The listing builds one solid part. Answer for the finished solid, in the listing's coordinates (mm). Face numbers are marked on the shaded views. A direction names the side the tool comes from. Round coordinates to 2 decimals unless told otherwise and drop trailing zeros. Loops run counter-clockwise (first coordinate to the right, second up) from the corner with the lowest first, then second, coordinate; pieces in that order, holes last. Notation, with made-up numbers: (30.25, 17.25) -> (76.25, 17.25) arc R17 ccw to (76.25, 38.25) -> close; hole circle Ø2 at (26.5, -15.5). An arc over 180 degrees is marked (long way). Answer in a Markdown table with one row per item. Add a question column.
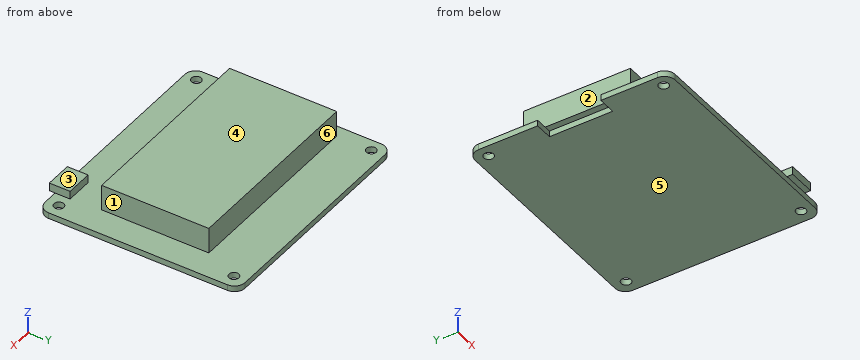
```python
from build123d import *

# Parameters (mm, degrees)
SKETCH_R     = 1.375
PAD_DEPTH    = 1.65
SKETCH001_W  = 54
SKETCH001_H  = 30
PAD001_DEPTH = 7.2
SKETCH002_W  = 7.57
SKETCH002_H  = 5.81
PAD002_DEPTH = 2.25


with BuildPart() as part:
    # Sketch (on Face4 of Binder) → Pad (new body)
    with BuildSketch(Plane.XY.offset(10.5)):
        with BuildLine():
            Line((-48.266962, 27.485719), (-48.266962, 10.985719))
            Line((-43.266962, 10.985719), (-48.266962, 10.985719))
            Line((-43.266962, -6.711357), (-43.266962, 10.985719))
            Line((-48.266962, -6.711357), (-43.266962, -6.711357))
            Line((-48.266962, -6.711357), (-48.266967, -22.514281))
            ThreePointArc((-48.266967, -22.514281), (-47.388287, -24.635602), (-45.266967, -25.514281))
            Line((-45.266967, -25.514281), (13.733038, -25.514281))
            ThreePointArc((13.733038, -25.514281), (15.854358, -24.635602), (16.733038, -22.514281))
            Line((16.733038, -22.514281), (16.733038, 27.485719))
            ThreePointArc((16.733038, 27.485719), (15.854358, 29.607039), (13.733038, 30.485719))
            Line((13.733038, 30.485719), (-45.266962, 30.485719))
            ThreePointArc((-45.266962, 30.485719), (-47.388282, 29.607039), (-48.266962, 27.485719))
        make_face()
        with Locations((-44.941962, 26.910719)):
            Circle(SKETCH_R, mode=Mode.SUBTRACT)
        with Locations((13.058038, 26.910719)):
            Circle(SKETCH_R, mode=Mode.SUBTRACT)
        with Locations((13.058038, -22.089281)):
            Circle(SKETCH_R, mode=Mode.SUBTRACT)
        with Locations((-44.941962, -22.089281)):
            Circle(SKETCH_R, mode=Mode.SUBTRACT)
    extrude(amount=PAD_DEPTH)

    # Sketch001 (on Face18 of Pad) → Pad001 (join)
    with BuildSketch(Plane.XY.offset(12.15)):
        with Locations((-18.066962, 2.137181)):
            Rectangle(SKETCH001_W, SKETCH001_H)
    extrude(amount=PAD001_DEPTH)

    # Sketch002 (on Face5 of Pad001) → Pad002 (join)
    with BuildSketch(Plane.XY.offset(12.15)):
        with Locations((5.748038, -24.209281)):
            Rectangle(SKETCH002_W, SKETCH002_H)
    extrude(amount=PAD002_DEPTH)


solid = part.part
```
Item 1: For the marked faces 1, 2 and 3, determine the directions among +Z, -Z, +X, -X, +Y, -Y from which every point of the face is accessible in a straight line to the end or side of a thin tool.
Item 2: Section A-A, the plane z = 13.5 is taken. Write down the section's boundary in (x, y).
Item 3: Section C-C, the plane y = 1 is taken. Write down the section's boundary in (x, z).
Item 4: Section B-B, the plane x = -38.5 is taken. Write down the section's boundary in (y, z), and give its area (3 significant figures).
Item 5: Flat-ended cylindrical pins translate along their axes: P1, Ø1, axis at x = 8, y = -21, coming from the +Z side; P2, Ø2, axis at y = 3.5, z = 18, coming from the -X side; P3, Ø1.8, axis at y = -24.5, z = 13.5, coming from the -X side; P4, Ø1.8, axis at x = 6.5, y = -26, coming from the -Z side. Find the tip coordinate at first contact, or state that the pin passes through.
Item 6: The mould has two halves that part along Z. Classify the marked faces 4, 5 and 6: +Z half, -Z half, draft (parallel to the pull), parting line (faces both ways), or undercut.
Item 7: Consider L1, parallel to Y at x = -23.5, z = 13; L2, parallel to Z at x = -42.5, y = -22.5; L3, parallel to X at y = 10, z = 11.25. Determine where each line is inside the solid, lowest interval first. Write a range as from..to.
Here are the results:
| question | item | result |
|---|---|---|
| 1 | face 1 | +Z, +X, +Y |
| 1 | face 2 | +Z, -X, +Y, -Y |
| 1 | face 3 | +Z, +X, -X, -Y |
| 2 | outline | (-45.07, -12.86) -> (8.93, -12.86) -> (8.93, 17.14) -> (-45.07, 17.14) -> close; (1.96, -27.11) -> (9.53, -27.11) -> (9.53, -21.3) -> (1.96, -21.3) -> close |
| 3 | outline | (-45.07, 12.15) -> (-43.27, 12.15) -> (-43.27, 10.5) -> (16.73, 10.5) -> (16.73, 12.15) -> (8.93, 12.15) -> (8.93, 19.35) -> (-45.07, 19.35) -> close |
| 4 | outline | (-25.51, 10.5) -> (30.49, 10.5) -> (30.49, 12.15) -> (17.14, 12.15) -> (17.14, 19.35) -> (-12.86, 19.35) -> (-12.86, 12.15) -> (-25.51, 12.15) -> close |
| 4 | area | 308 mm² |
| 5 | P1 | stops at z = 14.4 |
| 5 | P2 | stops at x = -45.07 |
| 5 | P3 | stops at x = 1.96 |
| 5 | P4 | stops at z = 10.5 |
| 6 | face 4 | +Z half |
| 6 | face 5 | -Z half |
| 6 | face 6 | draft |
| 7 | L1 | y = -12.86..17.14 |
| 7 | L2 | z = 10.5..12.15 |
| 7 | L3 | x = -43.27..16.73 |
